Verification items for the finished model (mm, model axes). Face numbers are marked on the shaded views. Round coordinates to 2 decimals unless told otherwise and drop trailing zeros. Write each loop counter-clockwise with the first axis right and the second up, starting at its lowest first coordinate (ties: lowest second). Pieces come first, ordered by that corner, then holes. Notation, with made-up numbers: M 9,89 L 57,89 A21 ccw 57,128 Z; hole C 13,42.25 d5. An arc over 180 degrees is marked long. Answer in a Markdown table with one row per item. Add a question column.
1. Material ranges on probe 1 along Y at (x, z) = (0, 8); probe 2 along Z at (x, y) = (3.25, 1.5); probe 3 along Y at (x, z) = (-1.25, 2.25), recorded low to high.
2. Sectioned sample at D-D on z = 9.5. Record the cut outline in (x, y).
3. Sectioned sample at C-C on z = 1.5. Record the cut outline in (x, y).
4. Draft check along X on the marked faces 1, 2 and 3. Enter one of: pulls with the +X half, pulls with the -X half, needs draft (parallel to the pull), parting line crosses it, or undercut.
5. Go/stop test with flat-tipped pins: pin 1 Ø3 at (x, y) = (-5, -2) entering from +Z; pin 2 Ø2 at (x, z) = (2, 1.5) entering from +Y; pin 3 Ø1 at (x, y) = (-4.5, -3.5) entering from -Z. Record where each tip stops, or that it passes through.
6. Sectioned sample at A-A on x = 0. Record the cut outline in (y, z).
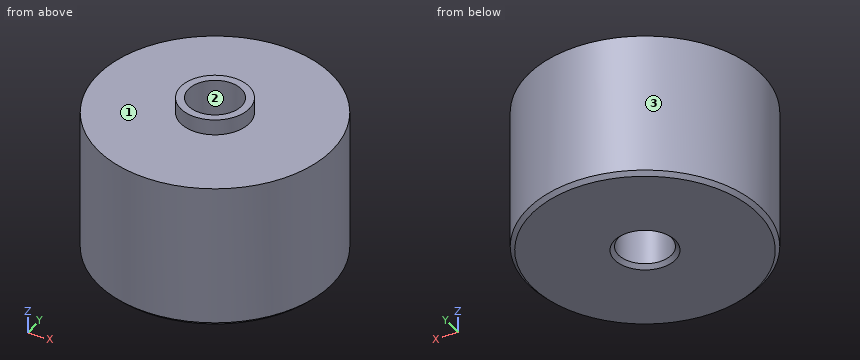
```python
from build123d import *

# Parameters (mm, degrees)
SKETCH1_R           = 7.5
SKETCH1_R_2         = 1.7
BOSS_EXTRUDE1_DEPTH = 9.3
SKETCH2_R           = 2.2
SKETCH2_R_2         = 1.7
BOSS_EXTRUDE2_DEPTH = 1
CHAMFER1_SIZE       = 0.25


with BuildPart() as part:
    # Sketch1 → Boss-Extrude1 (new body)
    with BuildSketch(Plane.XY):
        Circle(SKETCH1_R)
        Circle(SKETCH1_R_2, mode=Mode.SUBTRACT)
    extrude(amount=BOSS_EXTRUDE1_DEPTH)

    # Sketch2 → Boss-Extrude2 (add)
    with BuildSketch(Plane.XY.offset(9.3)):
        Circle(SKETCH2_R)
        Circle(SKETCH2_R_2, mode=Mode.SUBTRACT)
    extrude(amount=BOSS_EXTRUDE2_DEPTH)

    # Chamfer1
    chamfer1_edges = [part.edges().sort_by_distance(p)[0] for p in [
        (-7.5, 0, 0),
        (-1.7, 0, 0),
    ]]
    chamfer(chamfer1_edges, length=CHAMFER1_SIZE)


solid = part.part
```
Geometry check:
| question | item | result |
|---|---|---|
| 1 | probe 1 | y = -7.5 to -1.7, 1.7 to 7.5 |
| 1 | probe 2 | z = 0 to 9.3 |
| 1 | probe 3 | y = -7.4 to -1.15, 1.15 to 7.4 |
| 2 | outline | C 0,0 d4.4; hole C 0,0 d3.4 |
| 3 | outline | C 0,0 d15; hole C 0,0 d3.4 |
| 4 | face 1 | needs draft |
| 4 | face 2 | undercut |
| 4 | face 3 | parting line crosses it |
| 5 | pin 1 | stops at z = 9.3 |
| 5 | pin 2 | stops at y = 7.43 |
| 5 | pin 3 | stops at z = 0 |
| 6 | outline | M -7.5,0.25 L -7.25,0 L -1.95,0 L -1.7,0.25 L -1.7,10.3 L -2.2,10.3 L -2.2,9.3 L -7.5,9.3 Z; M 1.7,0.25 L 1.95,0 L 7.25,0 L 7.5,0.25 L 7.5,9.3 L 2.2,9.3 L 2.2,10.3 L 1.7,10.3 Z |
